```python
from build123d import *

# Parameters (mm, degrees)
SKETCH1_R           = 13.65
SKETCH1_R_2         = 12.15
BOSS_EXTRUDE1_DEPTH = 10
SKETCH1_4_R         = 12.15
SKETCH1_4_R_2       = 1.5
SKETCH1_4_R_3       = 4.25
BOSS_EXTRUDE2_DEPTH = 1.6
BOSS_EXTRUDE3_DEPTH = 9
SKETCH3_R           = 1.6
CUT_EXTRUDE1_DEPTH  = 18
CUT_EXTRUDE2_START  = 3
CUT_EXTRUDE2_DEPTH  = 16


with BuildPart() as part:
    # Sketch1 → Boss-Extrude1 (new body)
    with BuildSketch(Plane.XY):
        with Locations((0, 21.45)):
            Circle(SKETCH1_R)
        with Locations((0, 21.45)):
            Circle(SKETCH1_R_2, mode=Mode.SUBTRACT)
    extrude(amount=BOSS_EXTRUDE1_DEPTH)

    # Sketch1<4> → Boss-Extrude2 (add)
    with BuildSketch(Plane.XY):
        with Locations((0, 21.45)):
            Circle(SKETCH1_4_R)
        with Locations((-9.25, 21.45)):
            Circle(SKETCH1_4_R_2, mode=Mode.SUBTRACT)
        with Locations((9.25, 21.45)):
            Circle(SKETCH1_4_R_2, mode=Mode.SUBTRACT)
        with Locations((0, 21.45)):
            Circle(SKETCH1_4_R_3, mode=Mode.SUBTRACT)
    extrude(amount=BOSS_EXTRUDE2_DEPTH)

    # Sketch2 → Boss-Extrude3 (add)
    with BuildSketch(Plane.XY):
        with BuildLine():
            Line((-13.65, 21.45), (-13.65, 0))
            Line((-13.65, 0), (13.65, 0))
            Line((13.65, 0), (13.65, 21.45))
            ThreePointArc((13.65, 21.45), (0, 7.8), (-13.65, 21.45))
        make_face()
    extrude(amount=BOSS_EXTRUDE3_DEPTH)

    # Sketch3 → Cut-Extrude1 (cut)
    with BuildSketch(Plane(origin=(0, 0, 0), x_dir=(1, 0, 0), z_dir=(0, 1, 0))):
        with Locations(Location((-9.44, -5.108703369, 0), (0, 0, 90))):
            Circle(SKETCH3_R)
        with Locations(Location((9.44, -5.108703369, 0), (0, 0, 90))):
            Circle(SKETCH3_R)
    extrude(amount=CUT_EXTRUDE1_DEPTH, mode=Mode.SUBTRACT)

    # Sketch4 → Cut-Extrude2 (cut)
    with BuildSketch(Plane(origin=(0, 0, 0), x_dir=(1, 0, 0), z_dir=(0, 1, 0)).offset(CUT_EXTRUDE2_START)):
        Polygon((-7.837853003, -2.333703369), (-11.042146997, -2.333703369), (-12.644293994, -5.108703369), (-11.042146997, -7.883703369), (-7.837853003, -7.883703369), (-6.235706006, -5.108703369), align=None)
        Polygon((11.042146997, -2.333703369), (7.837853003, -2.333703369), (6.235706006, -5.108703369), (7.837853003, -7.883703369), (11.042146997, -7.883703369), (12.644293994, -5.108703369), align=None)
    extrude(amount=CUT_EXTRUDE2_DEPTH, mode=Mode.SUBTRACT)


solid = part.part
```
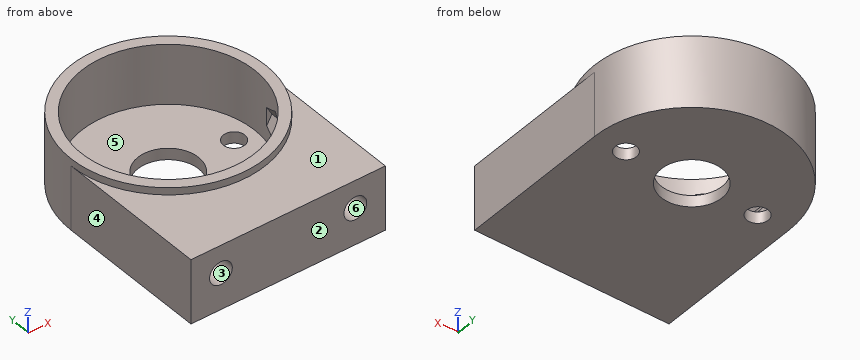
CAD build for the part. Positions are in the model's coordinates, mm. Face numbers are marked on the shaded views. A direction names the side the tool comes from. Round coordinates to 2 decimals unless told otherwise and drop trailing zeros. Write each loop counter-clockwise with the first axis right and the second up, starting at its lowest first coordinate (ties: lowest second). Pieces come first, ordered by that corner, then holes.
Item 1: Mould opens along Z. For the marked faces 1, 2 and 3 say: released by +Z, released by -Z, zero draft, split by the parting line, or undercut.
Filled in:
face 1: released by +Z
face 2: zero draft
face 3: undercut
Item 2: Tool access for the marked faces 4, 5 and 6: list every direction of +Z, -Z, +X, -X, +Y, -Y with a clear straight run to the whole face (end or side of a thin tool).
Filled in:
face 4: +Z, -Z, -X, +Y, -Y
face 5: +Z
face 6: -Y
Item 3: Band-saw the part on B-B on x = -9.44. Write the cut outline in (y, z).
Filled in:
outline: (0, 0) - (19.96, 0) - (19.96, 1.6) - (13.8, 1.6) - (13.8, 2.33) - (3, 2.33) - (3, 3.51) - (0, 3.51) - close; (0, 6.71) - (3, 6.71) - (3, 7.88) - (13.8, 7.88) - (13.8, 10) - (11.59, 10) - (11.59, 9) - (0, 9) - close; (22.94, 0) - (31.31, 0) - (31.31, 10) - (29.1, 10) - (29.1, 1.6) - (22.94, 1.6) - close
Item 4: Band-saw the part on D-D on x = -0.25. Write the cut outline in (y, z), then the cut area to 3 significant figures.
Filled in:
outline: (0, 0) - (17.21, 0) - (17.21, 1.6) - (9.3, 1.6) - (9.3, 10) - (7.8, 10) - (7.8, 9) - (0, 9) - close; (25.69, 0) - (35.1, 0) - (35.1, 10) - (33.6, 10) - (33.6, 1.6) - (25.69, 1.6) - close
area: 126 mm2
Item 5: Band-saw the part on A-A on y = 6.5. Write the cut outline in (x, z), then the cut area to 3 significant figures.
Filled in:
outline: (-13.65, 0) - (13.65, 0) - (13.65, 9) - (-13.65, 9) - close; hole (-12.64, 5.11) - (-11.04, 2.33) - (-7.84, 2.33) - (-6.24, 5.11) - (-7.84, 7.88) - (-11.04, 7.88) - close; hole (6.24, 5.11) - (7.84, 2.33) - (11.04, 2.33) - (12.64, 5.11) - (11.04, 7.88) - (7.84, 7.88) - close
area: 192 mm2
Item 6: Drill centre lines: L1, parallel to Z at x = 9.44, y = 1.7; L2, parallel to X at y = 4.5, z = 7.5; L3, parallel to Y at x = 0, z = 7. Where is each one in solid material? Low to high.
Filled in:
L1: z = 0 to 3.51, 6.71 to 9
L2: x = -13.65 to -11.26, -7.62 to 7.62, 11.26 to 13.65
L3: y = 0 to 9.3, 33.6 to 35.1
Item 7: Band-saw the part on C-C on y = 18. Write the cut outline in (x, z).
Filled in:
outline: (-13.65, 0) - (-2.48, 0) - (-2.48, 1.6) - (-11.65, 1.6) - (-11.65, 3.39) - (-12.64, 5.11) - (-11.65, 6.83) - (-11.65, 10) - (-13.21, 10) - (-13.21, 9) - (-13.65, 9) - close; (2.48, 0) - (13.65, 0) - (13.65, 9) - (13.21, 9) - (13.21, 10) - (11.65, 10) - (11.65, 6.83) - (12.64, 5.11) - (11.65, 3.39) - (11.65, 1.6) - (2.48, 1.6) - close
Item 8: Drop flat-ended pins along their axis: pin 1 Ø14.5 at (x, y) = (0, 21.45) entering from +Z; pin 2 Ø3 at (x, z) = (9.44, 5.11) entering from -Y; pin 3 Ø1.7 at (x, z) = (8.5, 5.5) entering from +Y; pin 4 Ø7.5 at (x, y) = (0, 21.45) entering from -Z. Give the stop position or say it passes through.
Filled in:
pin 1: stops at z = 1.6
pin 2: stops at y = 26.74
pin 3: stops at y = 32.75
pin 4: passes through
